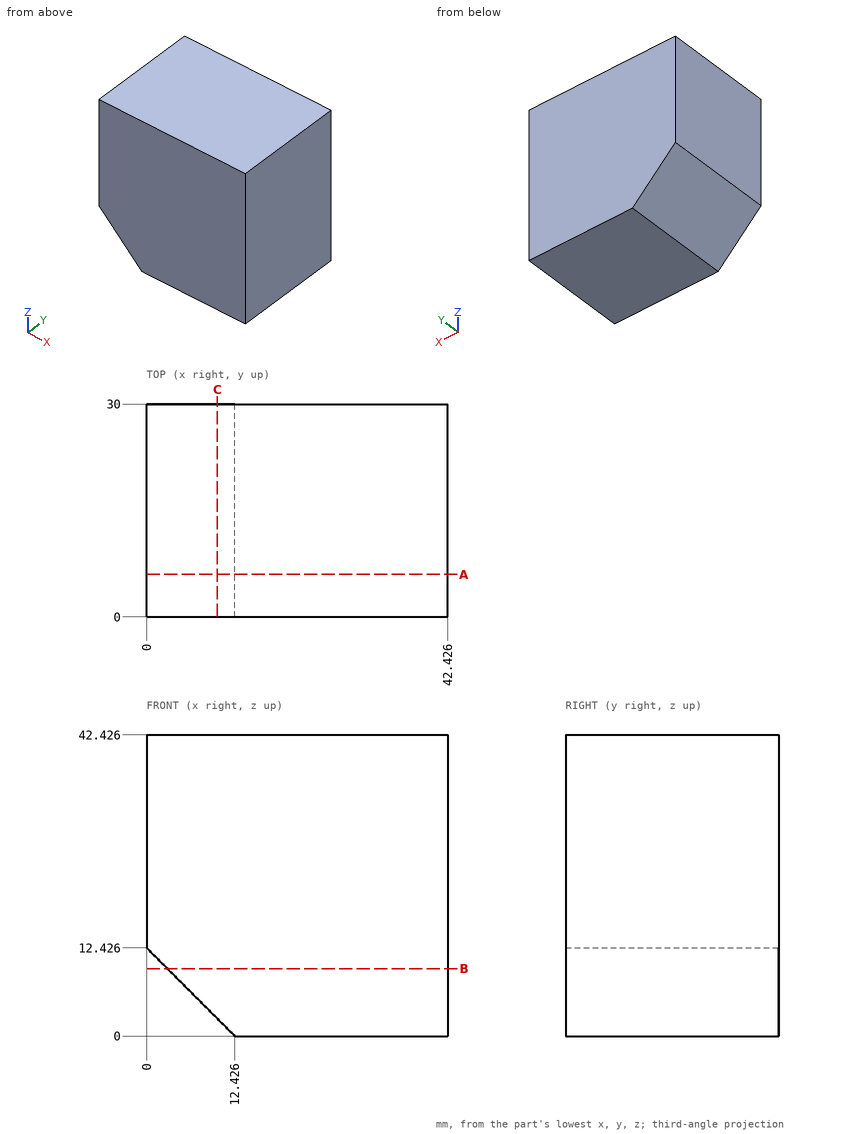
Check sheet for the drawn part. Datum: minimum x, y, z corner. Units: mm. Give positions to 0.01 mm unless a question says otherwise; leave off trailing zeros. Write each loop counter-clockwise with the first axis right and the second up, starting at its lowest first coordinate (ties: lowest second). Pieces come first, ordered by that corner, then holes. Notation, with made-up numbers: (-14, 9) -> (23, 9) arc R27 cw to (23, 30) -> close; hole circle Ø10 at (-24.5, 77). An arc over 180 degrees is marked (long way). Use one line per item in the form item = value. Start each with the question number.
1. Section check C-C (x = 10). Record the cut outline in (y, z), and give its area (3 significant figures).
2. Thickness scan on line 1 along X through (y, z) = (23, 4) (1 decimal); line 2 along X through (y, z) = (27.5, 6) (1 decimal); line 3 along Z through (x, y) = (11.5, 21.5) (1 decimal). Record the ranges inside material, lowest first. Write a range as from..to.
3. Go/stop test with a flat-tipped pin: P1, Ø3, axis at x = 7, y = 14.5, coming from the -Z side (1 decimal). Record where the tip stops, or that it passes through.
4. Section check B-B (z = 9.5). Record the cut outline in (x, y).
5. Section check A-A (y = 6). Record the cut outline in (x, z), and give its area (3 significant figures).
Conclusion:
q1.outline = (0, 2.43) -> (30, 2.43) -> (30, 42.43) -> (0, 42.43) -> close
q1.area = 1,200 mm²
q2.line_1 = 8.4..42.4
q2.line_2 = 6.4..42.4
q2.line_3 = 0.9..42.4
q3.P1 = 3.9
q4.outline = (2.93, 0) -> (42.43, 0) -> (42.43, 30) -> (2.93, 30) -> close
q5.outline = (0, 12.43) -> (12.43, 0) -> (42.43, 0) -> (42.43, 42.43) -> (0, 42.43) -> close
q5.area = 1,720 mm²
